Model file for the job. Use its own axes, mm. A direction names the side the tool comes from. Give positions to 0.01 mm unless a question says otherwise; leave off trailing zeros. Loops run counter-clockwise (first coordinate to the right, second up) from the corner with the lowest first, then second, coordinate; pieces in that order, holes last. Notation, with made-up numbers: M -2.5,-3 L 48.5,-3 A18 cw 48.5,31 Z; hole C 31.25,20 d3. An arc over 180 degrees is marked long. Use CSV: the item, a comma, the result in double quotes. Start each with the question number.
(1) Slice it at B-B on z = 1.7. List the corners of the cut face in (x, y), and give its area (3 significant figures).
(2) Wall check: line 1 along Y through (x, z) = (166.5, 2.35); line 2 along Y through (x, z) = (169.25, 0.65); line 3 along Y through (x, z) = (171.75, 2). Give the ranges that are in metal, low to high. Write a range as from..to.
(3) Slice it at A-A on x = 164. List the corners of the cut face in (y, z).
(4) Two-plate mould, pull along Y, no slides. Class faces 4 (the face through (156.845, -54.007, 1.479)), 5 (the face through (160.812, -58.393, 1.479)), 6 (the face through (168.09, -102.78, 1.48)): pulls with the +Y half, pulls with the -Y half, needs draft (parallel to the pull), parting line crosses it, or undercut.
(5) Tool access for faces 1 (the face through (175.423, -79.951, 1.479)), 2 (the face through (165.6, -98.18, 1.48)), 3 (the face through (165.422, -95.152, 1.479)): list every direction of +Z, -Z, +X, -X, +Y, -Y with a clear straight run to the whole face (end or side of a thin tool).
(6) Slice it at C-C on y = -89.5. List the corners of the cut face in (x, z).
(7) Slice it at D-D on x = 168.25. List the corners of the cut face in (y, z), and give its area (3 significant figures).
```python
from build123d import *

# Parameters (mm, degrees)
BASE_EXTRUDE_DEPTH = 3


with BuildPart() as part:
    # Sketch1 → Base-Extrude (new body)
    with BuildSketch(Plane.XY):
        Polygon((156.049697038, -56.981976311), (160.995963781, -94.739977013), (169.973055579, -95.576486697), (169.694713282, -98.563546383), (161.395541391, -97.790207109), (162.011434279, -102.491709341), (174.332527404, -103.072899505), (176.544882919, -56.17148924), (157.617642362, -51.114031919), align=None)
        Polygon((160.419784952, -59.862246689), (172.013048365, -62.960027094), (172.787493466, -60.061711241), (161.194230053, -56.963930836), align=None, mode=Mode.SUBTRACT)
    extrude(amount=BASE_EXTRUDE_DEPTH)


solid = part.part
```
Reply:
1,outline,"M 156.05,-56.98 L 161,-94.74 L 169.97,-95.58 L 169.69,-98.56 L 161.4,-97.79 L 162.01,-102.49 L 174.33,-103.07 L 176.54,-56.17 L 157.62,-51.11 Z; hole M 160.42,-59.86 L 172.01,-62.96 L 172.79,-60.06 L 161.19,-56.96 Z"
1,area,"756 mm^2"
2,line 1,"y = -102.7..-98.27, -95.25..-61.49, -58.38..-53.49"
2,line 2,"y = -102.83..-98.52, -95.51..-62.22, -59.12..-54.22"
2,line 3,"y = -102.95..-62.89, -59.78..-54.89"
3,outline,"M -102.59,0 L -98.03,0 L -98.03,3 L -102.59,3 Z; M -95.02,0 L -60.82,0 L -60.82,3 L -95.02,3 Z; M -57.71,0 L -52.82,0 L -52.82,3 L -57.71,3 Z"
4,face 4,"pulls with the +Y half"
4,face 5,"undercut"
4,face 6,"pulls with the -Y half"
5,face 1,"+Z, -Z, +X, -Y"
5,face 2,"+Z, -Z"
5,face 3,"+Z, -Z, -X"
6,outline,"M 160.31,0 L 174.97,0 L 174.97,3 L 160.31,3 Z"
7,outline,"M -102.79,0 L -98.43,0 L -98.43,3 L -102.79,3 Z; M -95.42,0 L -61.95,0 L -61.95,3 L -95.42,3 Z; M -58.85,0 L -53.96,0 L -53.96,3 L -58.85,3 Z"
7,area,"128 mm^2"
